```python
from build123d import *

# Parameters (mm, degrees)
F0_R      = 27.5
F1_DEPTH  = 50
F3_DEPTH  = 25
F4_W      = 25
F4_H      = 33.110834
F5_DEPTH  = 175
F7_DEPTH  = 25.4
F9_DEPTH  = 125
F10_W     = 115.094
F10_H     = 29.507754
F11_DEPTH = 25.4


with BuildPart() as f1:
    # F0 (on Right) → F1 (new body)
    with BuildSketch(Plane.YZ):
        with Locations((-5.465579, 22.014137)):
            Circle(F0_R)
    extrude(amount=F1_DEPTH)

    # F2 (on face) → F3 (join)
    with BuildSketch(Plane.YZ.offset(50)):
        with BuildLine():
            ThreePointArc((11.164121, 0.112013), (11.089932, 0.055881), (11.015554, 0))
            Line((11.015554, 0), (11.164121, 0))
            Line((11.164121, 0), (11.164121, 0.112013))
        make_face()
        with BuildLine():
            Line((-21.946713, 43.916262), (-21.946713, 0))
            Line((-21.946713, 0), (11.015554, 0))
            ThreePointArc((11.015554, 0), (11.089932, 0.055881), (11.164121, 0.112013))
            Line((11.164121, 0.112013), (11.164121, 43.916262))
            Line((11.164121, 43.916262), (-21.946713, 43.916262))
        make_face()
    extrude(amount=F3_DEPTH)

    # F4 (on face) → F5 (join)
    with BuildSketch(Plane.XY.offset(43.916262)):
        with Locations((62.5, -5.391296)):
            Rectangle(F4_W, F4_H)
    extrude(amount=F5_DEPTH)

    # F6 (on face) → F7 (join)
    with BuildSketch(Plane.YZ.offset(75)):
        with BuildLine():
            ThreePointArc((-21.946713, 198.658526), (-5.391296, 182.103109), (11.164121, 198.658526))
            ThreePointArc((11.164121, 198.658526), (-5.391296, 215.213943), (-21.946713, 198.658526))
        make_face()
    extrude(amount=F7_DEPTH)

    # F8 (on face) → F9 (join)
    with BuildSketch(Plane.YZ.offset(100.4)):
        with BuildLine():
            Line((-20.150423, 206.158526), (-55.391296, 206.158526))
            Line((-55.391296, 206.158526), (-55.391296, 191.158526))
            Line((-55.391296, 191.158526), (-20.150423, 191.158526))
            ThreePointArc((-20.150423, 191.158526), (-21.946713, 198.658526), (-20.150423, 206.158526))
        make_face()
        with BuildLine():
            Line((44.608704, 206.158526), (9.367831, 206.158526))
            ThreePointArc((9.367831, 206.158526), (10.708787, 202.514581), (11.164121, 198.658526))
            ThreePointArc((11.164121, 198.658526), (10.708787, 194.80247), (9.367831, 191.158526))
            Line((9.367831, 191.158526), (44.608704, 191.158526))
            Line((44.608704, 191.158526), (44.608704, 206.158526))
        make_face()
        with BuildLine():
            Line((9.367831, 206.158526), (-20.150423, 206.158526))
            ThreePointArc((-20.150423, 206.158526), (-21.946713, 198.658526), (-20.150423, 191.158526))
            Line((-20.150423, 191.158526), (9.367831, 191.158526))
            ThreePointArc((9.367831, 191.158526), (10.708787, 194.80247), (11.164121, 198.658526))
            ThreePointArc((11.164121, 198.658526), (10.708787, 202.514581), (9.367831, 206.158526))
        make_face()
    extrude(amount=F9_DEPTH)

    # F10 (on face) → F11 (cut)
    with BuildSketch(Plane.XY.offset(206.158526)):
        with Locations((157.947, -5.386046)):
            Rectangle(F10_W, F10_H)
    extrude(amount=-F11_DEPTH, mode=Mode.SUBTRACT)


solid = f1.part
```
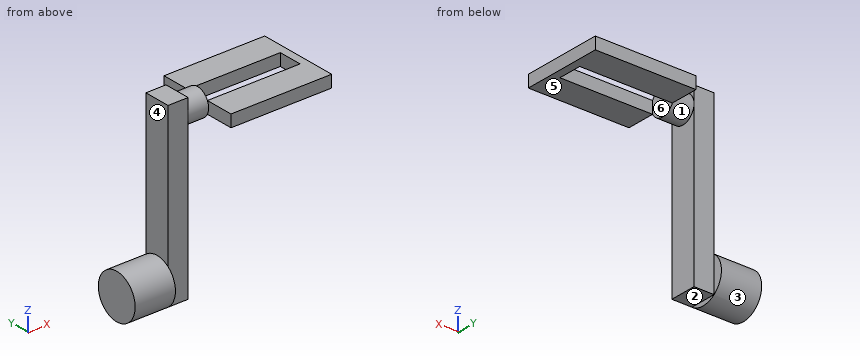
Geometry: final body of the model. Coordinates: model frame, mm. Face numbers are marked on the shaded views. A direction names the side the tool comes from. Round coordinates to 2 decimals unless told otherwise and drop trailing zeros. Loops run counter-clockwise (first coordinate to the right, second up) from the corner with the lowest first, then second, coordinate; pieces in that order, holes last. Notation, with made-up numbers: (-21.5, -6.5) -> (28.5, -6.5) arc R30 cw to (28.5, 19.5) -> close; hole circle Ø11 at (53.5, -18). An arc over 180 degrees is marked (long way). Use one line per item in the form item = value.
Item 1: Access query for the marked faces 1, 2 and 3. Directions: +Z, -Z, +X, -X, +Y, -Y. A direction counts if a zero-diameter tool reaches every point of the face in a straight line with its end or side. Return the directions, or none.
Evaluation:
face_1 = none
face_2 = -Z, +X, +Y, -Y
face_3 = -X
Item 2: Contact query for flat-ended pins moving along their axis: pin 1 Ø2 at (x, y) = (84, -18.5) entering from -Z; pin 2 Ø12 at (x, z) = (64, 28.5) entering from +Y; pin 3 Ø4 at (x, z) = (72.5, 68) entering from -Y; pin 4 Ø22.5 at (y, z) = (1.5, 213.5) entering from +X. Output: stop coordinate, or through.
Evaluation:
pin_1 = 187.37
pin_2 = 11.16
pin_3 = -21.95
pin_4 = 225.4
Item 3: Draft query along X for the marked faces 4, 5 and 6. Return one class per face: released by +X, released by -X, zero draft, split by the parting line, or undercut.
Evaluation:
face_4 = released by -X
face_5 = zero draft
face_6 = undercut
Item 4: Cut plane C-C on z = 38. Output: boundary loops of the cut face in (x, y).
Evaluation:
outline = (0, -27.84) -> (50, -27.84) -> (50, -21.95) -> (75, -21.95) -> (75, 11.16) -> (50, 11.16) -> (50, 16.91) -> (0, 16.91) -> close
Item 5: Cut plane B-B on y = -14.5. Output: boundary loops of the cut face in (x, z), then the cut area to 3 significant figures.
Evaluation:
outline = (0, -3.96) -> (50, -3.96) -> (50, 0) -> (75, 0) -> (75, 184.83) -> (100.4, 184.83) -> (100.4, 212.48) -> (75, 212.48) -> (75, 218.92) -> (50, 218.92) -> (50, 47.99) -> (0, 47.99) -> close; (215.49, 191.16) -> (225.4, 191.16) -> (225.4, 206.16) -> (215.49, 206.16) -> close
area = 8,920 mm2
Item 6: Cut plane D-D on y = -40.5. Output: boundary loops of the cut face in (x, z), then the cut area to 4 significant figures.
Evaluation:
outline = (100.4, 191.16) -> (225.4, 191.16) -> (225.4, 206.16) -> (100.4, 206.16) -> close
area = 1,875 mm2
Item 7: Cut plane A-A on x = 143. Output: boundary loops of the cut face in (y, z), then the cut area to 3 significant figures.
Evaluation:
outline = (-55.39, 191.16) -> (-20.14, 191.16) -> (-20.14, 206.16) -> (-55.39, 206.16) -> close; (9.37, 191.16) -> (44.61, 191.16) -> (44.61, 206.16) -> (9.37, 206.16) -> close
area = 1,060 mm2
Item 8: Material intervals for probe 1 along X at (y, z) = (4, 103); probe 2 along Z at (x, y) = (123.5, -25.5); probe 3 along X at (y, z) = (-5, 11.5), sorted ascending.
Evaluation:
probe_1 = 50 to 75
probe_2 = 191.16 to 206.16
probe_3 = 0 to 75
